from build123d import *

# Parameters (mm, degrees)
SKETCH1_W           = 95.25
SKETCH1_H           = 50.8
BOSS_EXTRUDE1_DEPTH = 12.7
SKETCH4_R           = 2.54
CUT_EXTRUDE3_DEPTH  = 64.816710194
FILLET2_R           = 2.54
SKETCH8_R           = 4.25
CUT_EXTRUDE4_DEPTH  = 6.35
SKETCH9_W           = 0.949786324
SKETCH9_H           = 5.291666667
CUT_EXTRUDE5_DEPTH  = 1.27
SKETCH10_R          = 3.937
CUT_EXTRUDE6_DEPTH  = 5.08


with BuildPart() as part:
    # Sketch1 → Boss-Extrude1 (new body)
    with BuildSketch(Plane(origin=(0, 0, 0), x_dir=(1, 0, 0), z_dir=(0, 1, 0))):
        with Locations((9.525, 0)):
            Rectangle(SKETCH1_W, SKETCH1_H)
    extrude(amount=BOSS_EXTRUDE1_DEPTH)

    # Sketch4 → Cut-Extrude3 (cut, through all)
    with BuildSketch(Plane(origin=(0, 12.7, 0), x_dir=(1, 0, 0), z_dir=(0, 1, 0))):
        with Locations(Location((-30.1625, 17.4625, 0), (0, 0, 270))):
            Circle(SKETCH4_R)
        with Locations(Location((49.2125, 17.4625, 0), (0, 0, 270))):
            Circle(SKETCH4_R)
        with Locations(Location((49.2125, -17.4625, 0), (0, 0, 270))):
            Circle(SKETCH4_R)
        with Locations(Location((-30.1625, -17.4625, 0), (0, 0, 270))):
            Circle(SKETCH4_R)
    extrude(amount=-CUT_EXTRUDE3_DEPTH, mode=Mode.SUBTRACT)

    # Fillet2
    fillet2_edges = [part.edges().sort_by_distance(p)[0] for p in [
        (57.15, 6.35, 25.4),
        (-38.1, 6.35, 25.4),
        (-38.1, 6.35, -25.4),
        (57.15, 6.35, -25.4),
    ]]
    fillet(fillet2_edges, radius=FILLET2_R)

    # Sketch6 → Cut-Revolve1 (revolve, cut)
    with BuildSketch(Plane.XY, mode=Mode.PRIVATE) as cut_revolve1_sk:
        Polygon((0, 0), (0, 12.7), (-16.129, 12.7), (-16.129, 3.65125), (-11.1125, 2.38125), (-11.1125, 0), align=None)
    revolve(cut_revolve1_sk.sketch.rotate(Axis((0, 0, 0), (0, 1, 0)), 180), axis=Axis((0, 0, 0), (0, 1, 0)), mode=Mode.SUBTRACT)

    # Sketch8 → Cut-Extrude4 (cut)
    with BuildSketch(Plane(origin=(0, 12.7, 0), x_dir=(1, 0, 0), z_dir=(0, 1, 0))):
        with Locations(Location((34.798, 0, 0), (0, 0, 270))):
            Circle(SKETCH8_R)
    extrude(amount=-CUT_EXTRUDE4_DEPTH, mode=Mode.SUBTRACT)

    # Sketch9 → Cut-Extrude5 (cut)
    # profile 1 of 7: a face of its own
    with BuildSketch(Plane.XY.offset(25.4)):
        Polygon((-12.727136752, 8.466666667), (-11.712688635, 8.466666667), (-10.35267094, 4.707802484), (-8.989473157, 8.466666667), (-7.978205128, 8.466666667), (-9.896858307, 3.175), (-10.811663662, 3.175), align=None)
    # profile 2 of 7: a face of its own
    with BuildSketch(Plane.XY.offset(25.4)):
        Polygon((-3.024687834, 8.466666667), (-2.143803419, 8.466666667), (-0.006784188, 3.175), (-1.021232305, 3.175), (-1.432523705, 4.260470085), (-3.738087607, 4.260470085), (-4.149379006, 3.175), (-5.162767094, 3.175), align=None)
        Polygon((-2.584775641, 7.047287326), (-3.377677618, 5.21025641), (-1.791873665, 5.21025641), align=None, mode=Mode.SUBTRACT)
    # profile 3 of 7: a face of its own
    with BuildSketch(Plane.XY.offset(25.4)):
        Polygon((3.249626068, 8.466666667), (4.105069778, 8.466666667), (6.506036325, 4.984470152), (6.506036325, 8.466666667), (7.45582265, 8.466666667), (7.45582265, 3.175), (6.594018763, 3.175), (4.199412393, 6.646596221), (4.199412393, 3.175), (3.249626068, 3.175), align=None)
    # profile 4 of 7: a face of its own
    with BuildSketch(Plane.XY.offset(25.4)):
        with Locations((11.49241453, 5.820833334)):
            Rectangle(SKETCH9_W, SKETCH9_H)
    # profile 5 of 7: a face of its own
    with BuildSketch(Plane.XY.offset(25.4)):
        Polygon((15.664690171, 8.466666667), (16.614476496, 8.466666667), (16.614476496, 4.124786325), (18.106997863, 4.124786325), (18.106997863, 3.175), (15.664690171, 3.175), align=None)
    # profile 6 of 7: a face of its own
    with BuildSketch(Plane.XY.offset(25.4)):
        Polygon((21.39732906, 8.466666667), (22.347115385, 8.466666667), (22.347115385, 4.124786325), (23.839636752, 4.124786325), (23.839636752, 3.175), (21.39732906, 3.175), align=None)
    # profile 7 of 7: a face of its own
    with BuildSketch(Plane.XY.offset(25.4)):
        Polygon((28.759233106, 8.466666667), (29.640117521, 8.466666667), (31.777136752, 3.175), (30.762688635, 3.175), (30.351397236, 4.260470085), (28.045833333, 4.260470085), (27.634541934, 3.175), (26.621153846, 3.175), align=None)
        Polygon((29.199145299, 7.047287326), (28.406243323, 5.21025641), (29.992047276, 5.21025641), align=None, mode=Mode.SUBTRACT)
    extrude(amount=-CUT_EXTRUDE5_DEPTH, mode=Mode.SUBTRACT)

    # Sketch10 → Cut-Extrude6 (cut)
    with BuildSketch(Plane(origin=(0, 12.7, 0), x_dir=(1, 0, 0), z_dir=(0, 1, 0))):
        with Locations(Location((-30.1625, 17.4625, 0), (0, 0, 270))):
            Circle(SKETCH10_R)
        with Locations(Location((-30.1625, -17.4625, 0), (0, 0, 270))):
            Circle(SKETCH10_R)
        with Locations(Location((49.2125, 17.4625, 0), (0, 0, 270))):
            Circle(SKETCH10_R)
        with Locations(Location((49.2125, -17.4625, 0), (0, 0, 270))):
            Circle(SKETCH10_R)
    extrude(amount=-CUT_EXTRUDE6_DEPTH, mode=Mode.SUBTRACT)


solid = part.part
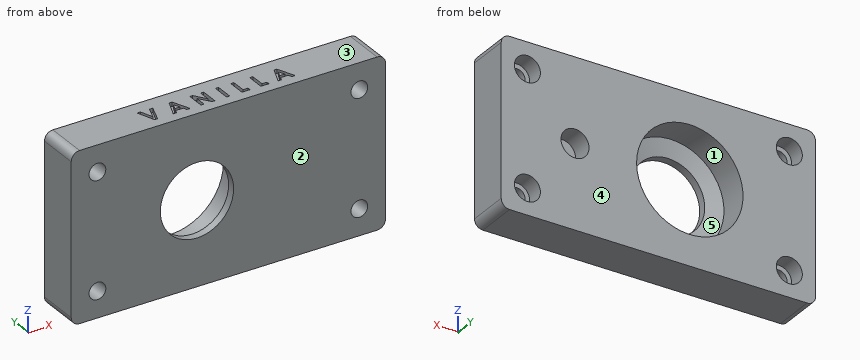
Can you work these out from the model? Positions are in its coordinate system, mm. Face numbers are marked on the shaded views. A direction names the side the tool comes from. Coordinates: 2 decimals unless noted, no trailing zeros. Loops run counter-clockwise (first coordinate to the right, second up) from the corner with the lowest first, then second, coordinate; pieces in that order, holes last. Notation, with made-up numbers: M 28,72.5 L 61,72.5 A18 cw 61,83.5 Z; hole C 72,64.25 d10. An arc over 180 degrees is marked long. Answer as CSV lines item,"result". Start each with the question number.
1. Suppose I cut it at A-A, the plane z = 0. List the corners of the cut face in (x, y) for me, plus the area to 3 significant figures.
2. For pin 1 Ø1.4 at (y, z) = (5.5, 25) entering from -X; pin 2 Ø5 at (x, z) = (34.798, 0) entering from +Y; pin 3 Ø1 at (y, z) = (6.5, 24.5) entering from +X, each with a flat end and sliding along its axis, tell me the tip position at first contact or that it passes through.
3. For the marked faces 1 and 2, which set-ups out of +Z, -Z, +X, -X, +Y, -Y let a thin tool reach every point of the face, with its end or its side?
4. If I drill on probe 1 along X at (y, z) = (3.5, -16); probe 2 along Z at (x, y) = (0, 1.8); probe 3 along Z at (x, y) = (51.5, 6), over which ranges is the centre line in solid material (lowest first)? Write a range as [from, to].
5. Thinking about a two-plate mould opening in Z: for the marked faces 3, 4 and 5, which applies, +Z half, -Z half, draft (parallel to the pull), parting line (faces both ways), or undercut?
Output:
1,outline,"M -38.1,0 L -11.11,0 L -11.11,2.38 L -16.13,3.65 L -16.13,12.7 L -38.1,12.7 Z; M 11.11,0 L 57.15,0 L 57.15,12.7 L 39.05,12.7 L 39.05,6.35 L 30.55,6.35 L 30.55,12.7 L 16.13,12.7 L 16.13,3.65 L 11.11,2.38 Z"
1,area,"776 mm^2"
2,pin 1,"stops at x = -37.65"
2,pin 2,"stops at y = 6.35"
2,pin 3,"stops at x = 56.88"
3,face 1,"+Y"
3,face 2,"+Z, -Z, +X, -X, -Y"
4,probe 1,"x = [-38.1, -32.24], [-28.09, 47.14], [51.29, 57.15]"
4,probe 2,"z = [-25.4, -11.11], [11.11, 25.4]"
4,probe 3,"z = [-25.4, -18.57], [-16.36, 16.36], [18.57, 25.4]"
5,face 3,"+Z half"
5,face 4,"draft"
5,face 5,"undercut"
